Autodesk Inventor part; units mm, degrees
ref_plane "YZ Plane" through (0, 0, 0) normal (1, 0, 0) x (0, 1, 0)
ref_plane "XZ Plane" through (0, 0, 0) normal (0, 1, 0) x (-1, 0, 0)
ref_plane "XY Plane" through (0, 0, 0) normal (0, 0, 1) x (1, 0, 0)
sketch "Sketch4" plane through (0, 0, 0) normal (0, 1, 0) x (1, 0, 0)
  line L0 (22.225, -12.319) -> (-22.225, -12.319) construction
  line L1 (0, 12.7356) -> (0, -16.4948) construction
  point P0 (0, 0)
  point P1 (22.225, 8.5598)
  point P2 (-22.225, 8.5598)
  dimension "d23" = 44.45
  dimension "d25" = 20.8788
  dimension "d26" = 12.319
sketch "Sketch1" plane through (0, 0, 0) normal (0, 1, 0) x (-1, 0, 0)
  line L0 (28.575, 18.669) -> (-28.575, 18.669)
  line L1 (-28.575, 18.669) -> (-28.575, 5.969)
  line L2 (-28.575, 5.969) -> (28.575, 5.969)
  line L3 (28.575, 5.969) -> (28.575, 18.669)
  line L4 (28.575, 18.669) -> (-28.575, 5.969) construction
  line L5 (-28.575, 18.669) -> (28.575, 5.969) construction
  line L6 (0, 3.429) -> (0, 21.209)
  point P0 (0, 12.319)
  point P1 (-22.225, 12.319)
  point P2 (0, 12.319)
  point P3 (0, 12.319)
  dimension "d27" = 6.35
  dimension "d28" = 6.35
  dimension "d29" = 6.35
extrude "Plate1" add sketch "Sketch1" along normal blind 0.9144
sketch "Sketch2" plane through (-28.575, 0.9144, 5.969) normal (0, -0.7071068, -0.7071068) x (1, 0, 0)
  line L0 (57.15, 0) -> (0, 0)
  line L1 (0, 0) -> (0, -6.8054)
  line L2 (0, -6.8054) -> (57.15, -6.8054)
  line L3 (57.15, -6.8054) -> (57.15, 0)
edge flange "Flange1" height 5.08 angle 45 thickness 0.9144 bend radius 0.762 thickness toward (0, -0.7071068, -0.7071068) relief tear relief width 0.9144 relief depth 0.4572 edges at (0, 0.9144, 5.969) wall of the first edge with corners at (28.575, 0.9144, 5.969) (-28.575, 0.9144, 5.969) (-28.575, 5.7266, 1.1568) (28.575, 5.7266, 1.1568)
bend "Bend1"
corner "Corner1"
sketch "Sketch3" plane through (28.575, 5.08, 0.5102) normal (0, 0.9961947, -0.0871557) x (-1, 0, 0)
  line L0 (57.15, 0) -> (0, 0)
  line L1 (0, 0) -> (0, -15.3978)
  line L2 (0, -15.3978) -> (57.15, -15.3978)
  line L3 (57.15, -15.3978) -> (57.15, 0)
edge flange "Flange2" height 15.8242 angle 50 thickness 0.9144 bend radius 0.762 thickness toward (0, 0.9961947, -0.0871557) relief tear relief width 0.9144 relief depth 0.4572 edges at (0, 5.08, 0.5102) wall of the first edge with corners at (-28.575, 5.08, 0.5102) (28.575, 5.08, 0.5102) (28.575, 3.738, -14.829) (-28.575, 3.738, -14.829)
bend "Bend2"
corner "Corner2"
hole "Hole1" at (22.225, 0, 12.319) at (-22.225, 0, 12.319) at (22.225, 0, -8.5598) at (-22.225, 0, -8.5598) direction (0, 1, 0) diameter 3.2512 end through all
fillet "Corner Round1" radius 6.35 4 edges at (28.575, 4.1935, -14.8688) (-28.575, 4.1935, -14.8688) (-28.575, 0.4572, 18.669) (28.575, 0.4572, 18.669)
equation "\"d35\" = Thickness"
equation "\"d2\" = Thickness"
equation "\"d3\" = BendReliefWidth"
equation "\"d4\" = BendReliefDepth"
equation "\"d5\" = MinimumRemnant"
equation "\"d6\" = TransitionRadius"
equation "\"d9\" = BendRadius"
equation "\"d10\" = CornerReliefSize"
equation "\"d11\" = GapSize"
equation "\"d12\" = JacobiRadiusSize"
equation "\"d13\" = BendReliefWidth"
equation "\"d14\" = BendReliefDepth"
equation "\"d15\" = MinimumRemnant"
equation "\"d16\" = TransitionRadius"
equation "\"d19\" = BendRadius"
equation "\"d20\" = CornerReliefSize"
equation "\"d21\" = GapSize"
equation "\"d22\" = JacobiRadiusSize"
equation "\"BendReliefWidth\" = Thickness"
equation "\"BendReliefDepth\" = 0.5 * Thickness"
equation "\"CornerReliefSize\" = 4 * Thickness"
equation "\"MinimumRemnant\" = 2 * Thickness"
equation "\"TransitionRadius\" = BendRadius"
equation "\"JacobiRadiusSize\" = BendRadius"
equation "\"GapSize\" = Thickness"
properties part number "J009836" material "STAINLESS STEEL, 316"
The listing builds one solid part. Answer for the finished solid, in the listing's coordinates (mm). A direction names the side the tool comes from. Coordinates: 2 decimals unless noted, no trailing zeros. Write each loop counter-clockwise with the first axis right and the second up, starting at its lowest first coordinate (ties: lowest second). Pieces come first, ordered by that corner, then holes. Notation, with made-up numbers: (84.5, 87.25) - (88.5, 87.25) arc R26 ccw to (88.5, 111.25) - close; hole circle Ø3 at (70, 26.5). An arc over 180 degrees is marked (long way). One line per item, written item: value.
1) Find section C-C (y = 2.4). Give the vertices of the cut face in (x, z) (3 decimals).
Geometry check:
outline: (-28.575, 3.19) - (28.575, 3.19) - (28.575, 4.483) - (-28.575, 4.483) - close
2) Find section A-A (x = -17). Give the vertices of the cut face in (y, z), and give its area (3 significant figures).
Geometry check:
outline: (0, 6.28) arc R1.68 ccw to (0.49, 5.1) - (4.83, 0.76) arc R0.76 cw to (5.05, 0.16) - (3.74, -14.83) - (4.65, -14.91) - (5.96, 0.08) arc R1.68 ccw to (5.48, 1.41) - (1.14, 5.75) arc R0.76 cw to (0.91, 6.28) - (0.91, 18.67) - (0, 18.67) - close
area: 32.5 mm2
3) Consider line 1 along Y through (x, z) = (-16, 8.5); line 2 along Z through (x, y) = (20.5, 0.5); line 3 along Y through (x, z) = (-26, 3.5). Determine where each line is inside the solid, lowest interval first. Write a range as from..to.
Geometry check:
line 1: y = 0..0.91
line 2: z = 5.09..18.67
line 3: y = 2.09..3.38
4) For a pull along X with two mould halves and no side action, classify faces 4 (the cylindrical face through (-0.4, 0.131, 5.635)), 5 (the cylindrical face through (-22.296, 0.464, 13.943)), 6 (the cylindrical face through (23.812, 0.464, 12.671)), 7 (the flat face through (28.575, 4, 2)) as pulls with the +X half, pulls with the -X half, needs draft (parallel to the pull), parting line crosses it, or undercut.
Geometry check:
face 4: needs draft
face 5: undercut
face 6: undercut
face 7: pulls with the +X half
5) A tool of negligible diameter and unlimited length cuts with its end or side. For faces 1 (the flat face through (0, 0.914, 13)), 2 (the flat face through (0, 0, 13)), 3 (the flat face through (-0.4, 2.69, 2.9)), from which of +Z, -Z, +X, -X, +Y, -Y can it reach the whole face along a straight path? Write none if from no direction.
Geometry check:
face 1: +Z, +X, -X, +Y
face 2: +Z, -Z, +X, -X, -Y
face 3: +X, -X, -Y
6) Each of these flat-tipped pins is pushed along its axis until it touches: pin 1 Ø10 at (x, z) = (-0.5, 10.5) entering from +Y; pin 2 Ø1 at (x, y) = (-4.5, 2.5) entering from +Z; pin 3 Ø4 at (x, z) = (22.22, -8.56) entering from -Y. Where does it stop, or does it pass through?
Geometry check:
pin 1: stops at y = 1.38
pin 2: stops at z = 4.88
pin 3: stops at y = 4.11
7) Find section B-B (z = 10). Give the vertices of the cut face in (x, y) (3 decimals), and give its area (3 significant figures).
Geometry check:
outline: (-28.575, 0) - (28.575, 0) - (28.575, 0.914) - (-28.575, 0.914) - close
area: 52.3 mm2
